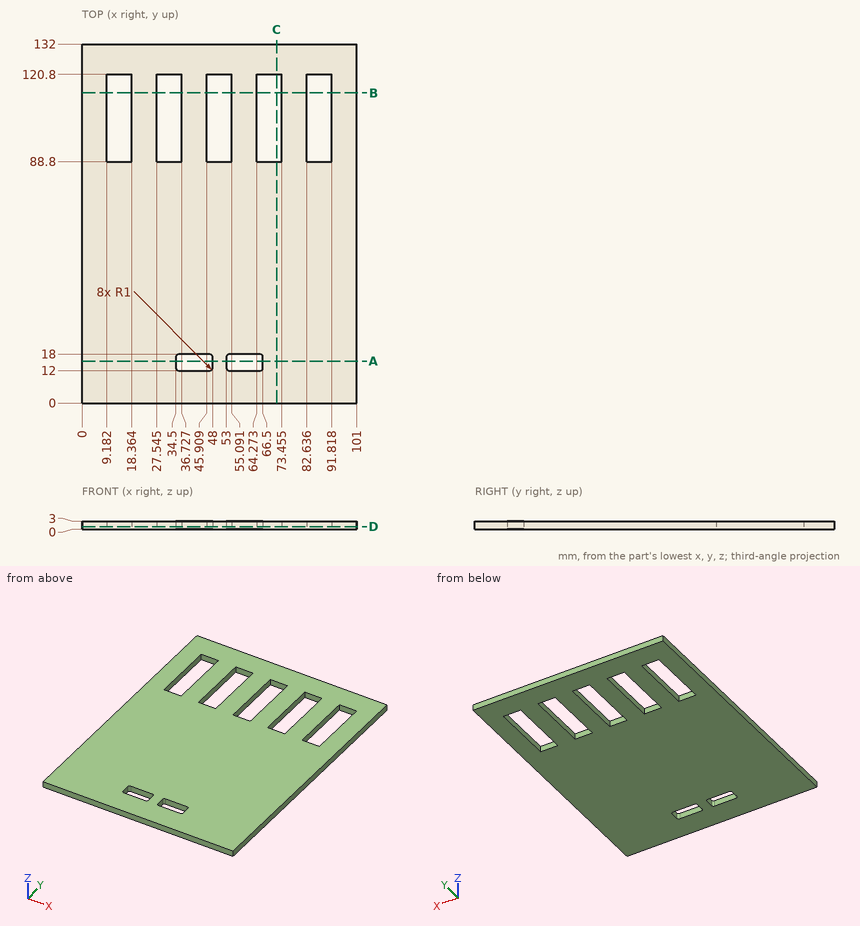
Could you check a few things on this drawing? It's one solid part, dimensions in mm from its lowest x, y, z. Give positions to 0.01 mm unless a question says otherwise; leave off trailing zeros. Loops run counter-clockwise (first coordinate to the right, second up) from the corner with the lowest first, then second, coordinate; pieces in that order, holes last. Notation, with made-up numbers: (54, 66.5) -> (101, 66.5) arc R20 cw to (101, 83.5) -> close; hole circle Ø5 at (-15, 34). An arc over 180 degrees is marked (long way). Use one line per item in the form item = value. Start each with the question number.
1) Imagine slicing it at D-D (z = 1). Count the separate pieces of the cut face and the enclosed holes in it, then the cut area to 3 significant figures.
2) For P1, Ø1.5, axis at y = 15.5, z = 1.5, coming from the -X side, with a flat end and sliding along its axis, tell me the tip position at first contact or that it passes through.
3) Imagine slicing it at A-A (y = 15.5). Please give me the cut outline in (x, z), then the cut area to 3 significant figures.
4) Imagine slicing it at C-C (x = 71.5). Please give me the cut outline in (y, z), then the cut area to 3 significant figures.
5) Please list where these lines run through material, in increasing order: line 1 along X through (y, z) = (13, 1.95); line 2 along Y through (x, z) = (64.5, 1.6); line 3 along Y through (x, z) = (28.5, 2.3).
6) Imagine slicing it at B-B (y = 114). Please give me the cut outline in (x, z) (1 decimal).
Check values:
q1.separate_pieces = 1
q1.enclosed_holes = 7
q1.area = 11,700 mm^2
q2.P1 = 0
q3.outline = (0, 0) -> (34.5, 0) -> (34.5, 3) -> (0, 3) -> close; (48, 0) -> (53, 0) -> (53, 3) -> (48, 3) -> close; (66.5, 0) -> (101, 0) -> (101, 3) -> (66.5, 3) -> close
q3.area = 222 mm^2
q4.outline = (0, 0) -> (88.8, 0) -> (88.8, 3) -> (0, 3) -> close; (120.8, 0) -> (132, 0) -> (132, 3) -> (120.8, 3) -> close
q4.area = 300 mm^2
q5.line_1 = 0 to 34.5, 48 to 53, 66.5 to 101
q5.line_2 = 0 to 12, 18 to 88.8, 120.8 to 132
q5.line_3 = 0 to 88.8, 120.8 to 132
q6.outline = (0, 0) -> (9.2, 0) -> (9.2, 3) -> (0, 3) -> close; (18.4, 0) -> (27.5, 0) -> (27.5, 3) -> (18.4, 3) -> close; (36.7, 0) -> (45.9, 0) -> (45.9, 3) -> (36.7, 3) -> close; (55.1, 0) -> (64.3, 0) -> (64.3, 3) -> (55.1, 3) -> close; (73.5, 0) -> (82.6, 0) -> (82.6, 3) -> (73.5, 3) -> close; (91.8, 0) -> (101, 0) -> (101, 3) -> (91.8, 3) -> close
